Check sheet for the modelled part. Datum: model origin and axes. Units: mm. A direction names the side the tool comes from. Round coordinates to 2 decimals unless told otherwise and drop trailing zeros. Loops run counter-clockwise (first coordinate to the right, second up) from the corner with the lowest first, then second, coordinate; pieces in that order, holes last. Notation, with made-up numbers: (-16, 81) -> (25, 81) arc R14 cw to (25, 86) -> close; hole circle Ø4 at (-30.75, 21.25). An arc over 180 degrees is marked (long way). One line per question, with ' | ' between items.
```python
from build123d import *

# Parameters (mm, degrees)
SKETCH1_R           = 9.5
BOSS_EXTRUDE1_DEPTH = 10
SKETCH2_R           = 12.5
BOSS_EXTRUDE2_DEPTH = 2
SKETCH3_R           = 5
BOSS_EXTRUDE3_DEPTH = 4
SKETCH4_R           = 12.5
SKETCH4_R_2         = 9.175
BOSS_EXTRUDE5_DEPTH = 4
SKETCH5_R           = 3
BOSS_EXTRUDE6_DEPTH = 10


with BuildPart() as part:
    # Sketch1 → Boss-Extrude1 (new body)
    with BuildSketch(Plane.XY):
        with BuildLine():
            Line((20, 6.21521961), (25, 6.21521961))
            Line((25, 6.21521961), (25, -6.21521961))
            Line((25, -6.21521961), (20, -6.21521961))
            add(Edge.make_bspline(
                [(20, -6.21521961), (14.928036397, -6.21521961), (10.891454701, -7.892862666), (6.69762749, -10.554230716)],
                knots=[0, 0, 0, 0, 1, 1, 1, 1], degree=3))
            ThreePointArc((6.69762749, -10.554230716), (-12.5, 0), (6.69762749, 10.554230716))
            add(Edge.make_bspline(
                [(20, 6.21521961), (14.928036397, 6.21521961), (10.891454701, 7.892862666), (6.69762749, 10.554230716)],
                knots=[0, 0, 0, 0, 1, 1, 1, 1], degree=3))
        make_face()
        Circle(SKETCH1_R, mode=Mode.SUBTRACT)
    extrude(amount=BOSS_EXTRUDE1_DEPTH)

    # Sketch2 → Boss-Extrude2 (add)
    with BuildSketch(Plane(origin=(0, 0, 0), x_dir=(-1, 0, 0), z_dir=(0, 0, -1))):
        Circle(SKETCH2_R)
    extrude(amount=-BOSS_EXTRUDE2_DEPTH)

    # Sketch3 → Boss-Extrude3 (add)
    with BuildSketch(Plane(origin=(0, 0, 0), x_dir=(-1, 0, 0), z_dir=(0, 0, -1))):
        Circle(SKETCH3_R)
    extrude(amount=-BOSS_EXTRUDE3_DEPTH)

    # Sketch4 → Boss-Extrude5 (add)
    with BuildSketch(Plane(origin=(0, 0, 0), x_dir=(-1, 0, 0), z_dir=(0, 0, -1))):
        Circle(SKETCH4_R)
        Circle(SKETCH4_R_2, mode=Mode.SUBTRACT)
    extrude(amount=-BOSS_EXTRUDE5_DEPTH)

    # Sketch5 → Boss-Extrude6 (add)
    with BuildSketch(Plane(origin=(25, 0, 0), x_dir=(0, 0, -1), z_dir=(1, 0, 0))):
        with Locations((-5, 0)):
            Circle(SKETCH5_R)
    extrude(amount=BOSS_EXTRUDE6_DEPTH)


solid = part.part
```
(1) Mould release check, pull along X, two halves, no side actions. Record for faces 5 (the face through (-8.75, 2.76, 2.99)), 6 (the face through (25, 3, 4)), 7 (the face through (29.93, 0.9, 2.14)): +X half, -X half, draft (parallel to the pull), parting line (faces both ways), or undercut.
Answer:
face 5: undercut | face 6: +X half | face 7: draft
(2) Scan lines: probe 1 along Y at (x, z) = (0, 2.5) (3 decimals); probe 2 along X at (y, z) = (0, 7.9); probe 3 along Y at (x, z) = (0, 6.9). Record each from-to range of solid material in increasing order.
Answer:
probe 1: y = -12.5 to -9.175, -5 to 5, 9.175 to 12.5 | probe 2: x = -12.5 to -9.5, 9.5 to 35 | probe 3: y = -12.5 to -9.5, 9.5 to 12.5
(3) Go/stop test with flat-tipped pins: pin 1 (11 mm diameter, centred on x = -1.5, y = 0, fed in from +Z); pin 2 (1 mm diameter, centred on y = -4, z = 8, fed in from +X); pin 3 (6 mm diameter, centred on y = -4.5, z = 4.5, fed in from +X); pin 4 (4 mm diameter, centred on x = 21.5, z = 5, fed in from +Y). Record where each tip stops, or that it passes through.
Answer:
pin 1: stops at z = 4 | pin 2: stops at x = 25 | pin 3: stops at x = 35 | pin 4: stops at y = 6.22
(4) Sectioned sample at A-A, the plane x = 0. Record the cut outline in (y, z) (3 decimals).
Answer:
outline: (-12.5, 0) -> (12.5, 0) -> (12.5, 10) -> (9.5, 10) -> (9.5, 4) -> (9.175, 4) -> (9.175, 2) -> (5, 2) -> (5, 4) -> (-5, 4) -> (-5, 2) -> (-9.175, 2) -> (-9.175, 4) -> (-9.5, 4) -> (-9.5, 10) -> (-12.5, 10) -> close
(5) Sectioned sample at D-D, the plane y = 5.75. Record the cut outline in (x, z), and give its area (3 significant figures).
Answer:
outline: (-11.1, 0) -> (25, 0) -> (25, 10) -> (7.56, 10) -> (7.56, 4) -> (7.15, 4) -> (7.15, 2) -> (-7.15, 2) -> (-7.15, 4) -> (-7.56, 4) -> (-7.56, 10) -> (-11.1, 10) -> close | area: 242 mm2
(6) Sectioned sample at C-C, the plane x = -6. Record the cut outline in (y, z).
Answer:
outline: (-10.97, 0) -> (10.97, 0) -> (10.97, 10) -> (7.37, 10) -> (7.37, 4) -> (6.94, 4) -> (6.94, 2) -> (-6.94, 2) -> (-6.94, 4) -> (-7.37, 4) -> (-7.37, 10) -> (-10.97, 10) -> close
(7) Set-up check for faces 1 (the face through (23, -6.215, 5)), 2 (the face through (35, 0, 5)), 3 (the face through (4.38, -8.43, 6.96)), 4 (the face through (22, 6.215, 5)): record each of +Z, -Z, +X, -X, +Y, -Y from which the full face is reachable in a straight line by a thin tool's end or side.
Answer:
face 1: +Z, -Z, +X, -Y | face 2: +Z, -Z, +X, +Y, -Y | face 3: +Z | face 4: +Z, -Z, +X, +Y
(8) Sectioned sample at B-B, the plane y = 0. Record the cut outline in (x, z) (3 decimals), and give its area (3 significant figures).
Answer:
outline: (-12.5, 0) -> (25, 0) -> (25, 2) -> (35, 2) -> (35, 8) -> (25, 8) -> (25, 10) -> (9.5, 10) -> (9.5, 4) -> (9.175, 4) -> (9.175, 2) -> (5, 2) -> (5, 4) -> (-5, 4) -> (-5, 2) -> (-9.175, 2) -> (-9.175, 4) -> (-9.5, 4) -> (-9.5, 10) -> (-12.5, 10) -> close | area: 304 mm2
